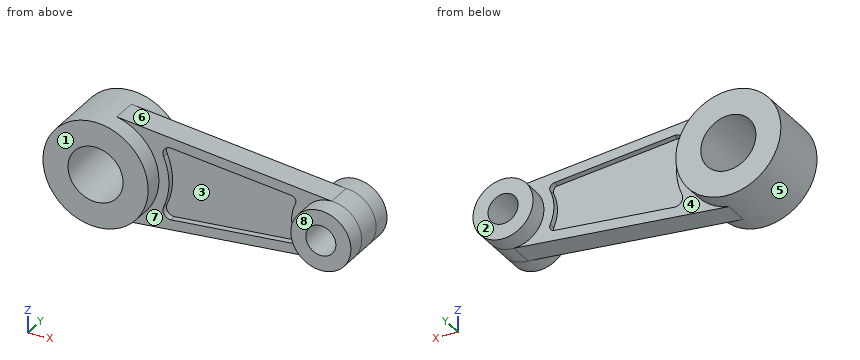
```python
from build123d import *
from build123d.topology import SkipClean

# Parameters (mm, degrees)
BOSS_EXTRUDE1_DEPTH = 10
SKETCH2_R           = 21
SKETCH2_R_2         = 12
BOSS_EXTRUDE2_DEPTH = 17.5
BOSS_EXTRUDE3_START = 7.5
SKETCH3_R           = 21
SKETCH3_R_2         = 12
BOSS_EXTRUDE3_DEPTH = 7.5
SKETCH4_R           = 11
SKETCH4_R_2         = 6
CUT_EXTRUDE1_DEPTH  = 38.5
CUT_EXTRUDE2_DEPTH  = 2.5
CUT_EXTRUDE3_START  = -2.5
CUT_EXTRUDE3_DEPTH  = 2.5


with BuildPart() as part:
    # Sketch1 → Boss-Extrude1 (new body)
    with BuildSketch(Plane(origin=(0, 0, 0), x_dir=(1, 0, 0), z_dir=(0, 1, 0))):
        with BuildLine():
            Line((0, 21), (90, 12))
            ThreePointArc((90, 12), (102, 0), (90, -12))
            Line((90, -12), (0, -21))
            ThreePointArc((0, -21), (-21, 0), (0, 21))
        make_face()
    extrude(amount=-BOSS_EXTRUDE1_DEPTH)

    # Sketch2 → Boss-Extrude2 (add)
    with SkipClean():  # the faces are left unmerged after this step: merging them gives an invalid solid
        with BuildSketch(Plane(origin=(0, 0, 0), x_dir=(1, 0, 0), z_dir=(0, 1, 0))):
            with Locations(Location((0, 0, 0), (0, 0, 270))):
                Circle(SKETCH2_R)
            with Locations(Location((90, 0, 0), (0, 0, 270))):
                Circle(SKETCH2_R_2)
        extrude(amount=-BOSS_EXTRUDE2_DEPTH)

    # Sketch3 → Boss-Extrude3 (add)
    with SkipClean():  # the faces are left unmerged after this step: merging them gives an invalid solid
        with BuildSketch(Plane(origin=(0, 0, 0), x_dir=(1, 0, 0), z_dir=(0, 1, 0)).offset(BOSS_EXTRUDE3_START)):
            with Locations(Location((0, 0, 0), (0, 0, 270))):
                Circle(SKETCH3_R)
            with Locations(Location((90, 0, 0), (0, 0, 270))):
                Circle(SKETCH3_R_2)
        extrude(amount=-BOSS_EXTRUDE3_DEPTH)

    # Sketch4 → Cut-Extrude1 (cut)
    with SkipClean():  # the faces are left unmerged after this step: merging them gives an invalid solid
        with BuildSketch(Plane(origin=(0, 7.5, 0), x_dir=(1, 0, 0), z_dir=(0, 1, 0))):
            with Locations(Location((0, 0, 0), (0, 0, 270))):
                Circle(SKETCH4_R)
            with Locations(Location((90, 0, 0), (0, 0, 270))):
                Circle(SKETCH4_R_2)
        extrude(amount=-CUT_EXTRUDE1_DEPTH, mode=Mode.SUBTRACT)

    # Sketch5 → Cut-Extrude2 (cut)
    with SkipClean():  # the faces are left unmerged after this step: merging them gives an invalid solid
        with BuildSketch(Plane(origin=(0, 0, 0), x_dir=(1, 0, 0), z_dir=(0, 1, 0))):
            with BuildLine():
                Line((25.869138462, 14.393135905), (73.882928765, 9.591756875))
                ThreePointArc((73.882928765, 9.591756875), (75.42197475, 8.591212838), (75.496818958, 6.757051106))
                ThreePointArc((75.496818958, 6.757051106), (74, 0), (75.496818958, -6.757051106))
                ThreePointArc((75.496818958, -6.757051106), (75.42197475, -8.591212838), (73.882928765, -9.591756875))
                Line((73.882928765, -9.591756875), (25.869138462, -14.393135905))
                ThreePointArc((25.869138462, -14.393135905), (23.13846438, -13.164322574), (22.830917237, -10.185736013))
                ThreePointArc((22.830917237, -10.185736013), (25, 0), (22.830917237, 10.185736013))
                ThreePointArc((22.830917237, 10.185736013), (23.13846438, 13.164322574), (25.869138462, 14.393135905))
            make_face()
        extrude(amount=-CUT_EXTRUDE2_DEPTH, mode=Mode.SUBTRACT)

    # Sketch7 → Cut-Extrude3 (cut)
    with SkipClean():  # the faces are left unmerged after this step: merging them gives an invalid solid
        with BuildSketch(Plane.XZ.offset(10).offset(CUT_EXTRUDE3_START)):
            with BuildLine():
                Line((25.869138462, 14.393135905), (73.882928765, 9.591756875))
                ThreePointArc((73.882928765, 9.591756875), (75.42197475, 8.591212838), (75.496818958, 6.757051106))
                ThreePointArc((75.496818958, 6.757051106), (74, 0), (75.496818958, -6.757051106))
                ThreePointArc((75.496818958, -6.757051106), (75.42197475, -8.591212838), (73.882928765, -9.591756875))
                Line((73.882928765, -9.591756875), (25.869138462, -14.393135905))
                ThreePointArc((25.869138462, -14.393135905), (23.13846438, -13.164322574), (22.830917237, -10.185736013))
                ThreePointArc((22.830917237, -10.185736013), (25, 0), (22.830917237, 10.185736013))
                ThreePointArc((22.830917237, 10.185736013), (23.13846438, 13.164322574), (25.869138462, 14.393135905))
            make_face()
        extrude(amount=CUT_EXTRUDE3_DEPTH, mode=Mode.SUBTRACT)


solid = part.part
```
Part model, mm, in its own coordinate system. Face numbers are marked on the shaded views. A direction names the side the tool comes from. Give positions to 0.01 mm unless a question says otherwise; leave off trailing zeros. Write each loop counter-clockwise with the first axis right and the second up, starting at its lowest first coordinate (ties: lowest second). Pieces come first, ordered by that corner, then holes. Notation, with made-up numbers: (79.25, 61) -> (87.25, 61) arc R17 ccw to (87.25, 82) -> close; hole circle Ø10 at (84.5, 28.5). An arc over 180 degrees is marked (long way). Put each result on its own line as item: value. Start each with the question number.
Item 1: Cut at D-D (y = -4.5). List the corners of the cut face in (x, z).
Item 2: Wall check: L1, parallel to X at y = -10.5, z = 0; L2, parallel to X at y = -3.75, z = 0; L3, parallel to X at y = -8, z = 6.5. Give the ranges that are in metal, low to high. Write a range as [from, to].
Item 3: Which spindle directions (+Z, -Z, +X, -X, +Y, -Y) get a long thin tool onto all of the face, cutting with end or side? Do the marked faces 1, 2, 3, 4 and 5. Say none if no direction does.
Item 4: Cut at C-C (x = -3). List the corners of the cut face in (y, z), then the cut area to 3 significant figures.
Item 5: Pin check, flat tips, straight feed: pin 1 Ø4 at (x, z) = (57, -9) entering from -Y; pin 2 Ø5 at (y, z) = (-14, -12) entering from -X; pin 3 Ø10 at (y, z) = (-2, 2.5) entering from -X. Stop position of each tip, or through.
Item 6: Cut at B-B (y = -12.5). List the corners of the cut face in (x, z).
Item 7: Cut at A-A (z = 0). List the corners of the cut face in (x, y).
Item 8: Pull direction X, two halves, no side cores. Call the marked faces 6, 7 and 8: pulls with the +X half, pulls with the -X half, needs draft (parallel to the pull), parting line crosses it, or undercut.
Answer list:
1. outline: (4.16, -20.58) -> (90, -12) arc R12 ccw to (90, 12) -> (4.16, 20.58) arc R21 ccw (long way) to start; hole circle Ø22 at (0, 0); hole circle Ø12 at (90, 0)
2. L1: x = [-21, -11], [11, 21], [78, 84], [96, 102]
2. L2: x = [-21, -11], [11, 84], [96, 102]
2. L3: x = [-19.97, -8.87], [8.87, 24.14], [75.38, 100.09]
3. face 1: +Z, -Z, +X, -X, -Y
3. face 2: +Z, -Z, +X, -X, +Y
3. face 3: -Y
3. face 4: +Y
3. face 5: none
4. outline: (-17.5, -20.78) -> (7.5, -20.78) -> (7.5, -10.58) -> (-17.5, -10.58) -> close; (-17.5, 10.58) -> (7.5, 10.58) -> (7.5, 20.78) -> (-17.5, 20.78) -> close
4. area: 510 mm2
5. pin 1: stops at y = -7.5
5. pin 2: stops at x = -18.73
5. pin 3: stops at x = -21
6. outline: circle Ø42 at (0, 0); circle Ø24 at (90, 0); hole circle Ø22 at (0, 0); hole circle Ø12 at (90, 0)
7. outline: (-21, -17.5) -> (-11, -17.5) -> (-11, 7.5) -> (-21, 7.5) -> close; (11, -17.5) -> (21, -17.5) -> (21, -10) -> (25, -10) -> (25, -7.5) -> (74, -7.5) -> (74, -10) -> (78, -10) -> (78, -17.5) -> (84, -17.5) -> (84, 7.5) -> (78, 7.5) -> (78, 0) -> (74, 0) -> (74, -2.5) -> (25, -2.5) -> (25, 0) -> (21, 0) -> (21, 7.5) -> (11, 7.5) -> close; (96, -17.5) -> (102, -17.5) -> (102, 7.5) -> (96, 7.5) -> close
8. face 6: pulls with the +X half
8. face 7: undercut
8. face 8: needs draft
